The listing builds one solid part. Answer for the finished solid, in the listing's coordinates (mm). Round coordinates to 2 decimals unless told otherwise and drop trailing zeros. Order: outer loops, then holes, each group sorted by start corner. A loop starts at its lowest first (then second) coordinate and runs counter-clockwise, first axis right, second up. Notation, with made-up numbers: M 43.25,-12 L 52.25,-12 A19 cw 52.25,-4 Z; hole C -33,87.5 d3. An arc over 180 degrees is marked long. Put each result on its own line as item: value. Start each with the question number.
1. The part is cut by section D-D (y = -11). Give the vertices of the cut face in (x, z).
2. The part is cut by section A-A (x = -17.5). Give the vertices of the cut face in (y, z).
3. Each of these flat-tipped pins is pushed along its axis until it touches: pin 1 Ø2 at (y, z) = (6, 3.5) entering from -X; pin 2 Ø4 at (y, z) = (4, 6) entering from +X; pin 3 Ø1.1 at (y, z) = (-31, 2.5) entering from +X; pin 4 Ø1.6 at (x, z) = (-2.5, 1.5) entering from +Y. Where does it stop, or does it pass through?
4. The part is cut by section C-C (x = 5). Give the vertices of the cut face in (y, z), then the cut area to 3 significant figures.
5. The part is cut by section B-B (y = -27). Give the vertices of the cut face in (x, z), then the cut area to 3 significant figures.
6. Consider line 1 (Y direction, x = -5, z = 1); line 2 (Y direction, x = 40.48, z = 2.2); line 3 (X direction, y = -54.5, z = 2.25). Determine where each line is inside the solid, lowest interval first.
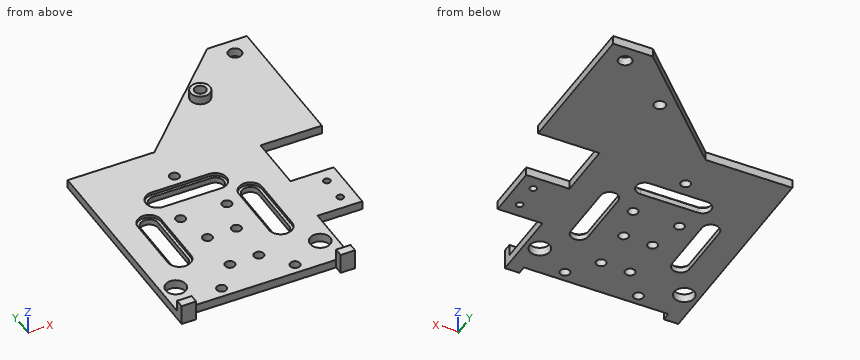
from build123d import *

# Parameters (mm, degrees)
SKETCH_R        = 2.3
SKETCH_R_2      = 1.7
SKETCH_R_3      = 1.2
PAD_DEPTH       = 3
SKETCH004_R     = 2.345013
SKETCH004_R_2   = 1.7
POCKET004_DEPTH = 5
SKETCH003_R     = 3.5
SKETCH003_R_2   = 2
POCKET005_DEPTH = 5
SKETCH005_R     = 3.4
PAD001_DEPTH    = 3
SKETCH006_R     = 2
POCKET_DEPTH    = 8
SKETCH009_R     = 2
POCKET007_DEPTH = 3
POCKET008_DEPTH = 1
SKETCH011_W     = 5
SKETCH011_H     = 3
PAD003_DEPTH    = 3
SKETCH012_W     = 5
SKETCH012_H     = 3
PAD004_DEPTH    = 4


with BuildPart() as part:
    # Sketch → Pad (new body)
    with BuildSketch(Plane.XY):
        Polygon((30, -63), (-30, -63), (-30, 10), (0, 10), (38, 48), (51.73, 48), (51.73, -2), (30.48, -2), (30.48, -22), (45.48, -22), (45.48, -41), (30, -41), align=None)
        with Locations((44.585025, 42.218019)):
            Circle(SKETCH_R, mode=Mode.SUBTRACT)
        with Locations((-12.71, -59.3)):
            Circle(SKETCH_R_2, mode=Mode.SUBTRACT)
        with Locations((12.71, -59.3)):
            Circle(SKETCH_R_2, mode=Mode.SUBTRACT)
        with Locations((0, -3.331213)):
            Circle(SKETCH_R_2, mode=Mode.SUBTRACT)
        with Locations((-8, -22.917882)):
            Circle(SKETCH_R_2, mode=Mode.SUBTRACT)
        with Locations((8, -22.917882)):
            Circle(SKETCH_R_2, mode=Mode.SUBTRACT)
        with Locations((40.48, -27)):
            Circle(SKETCH_R_3, mode=Mode.SUBTRACT)
        with Locations((40.48, -36)):
            Circle(SKETCH_R_3, mode=Mode.SUBTRACT)
        with Locations((-5, -35)):
            Circle(SKETCH_R_2, mode=Mode.SUBTRACT)
        with Locations((5, -35)):
            Circle(SKETCH_R_2, mode=Mode.SUBTRACT)
        with Locations((-5, -50)):
            Circle(SKETCH_R_2, mode=Mode.SUBTRACT)
        with Locations((5, -50)):
            Circle(SKETCH_R_2, mode=Mode.SUBTRACT)
        with BuildLine():
            ThreePointArc((-20.5, -40.385975), (-17.5, -43.385975), (-14.5, -40.385975))
            Line((-14.5, -40.385975), (-14.5, -20.385975))
            ThreePointArc((-14.5, -20.385975), (-17.5, -17.385975), (-20.5, -20.385975))
            Line((-20.5, -40.385975), (-20.5, -20.385975))
        make_face(mode=Mode.SUBTRACT)
        with BuildLine():
            ThreePointArc((14.5, -40.385975), (17.5, -43.385975), (20.5, -40.385975))
            Line((20.5, -40.385975), (20.5, -20.385975))
            ThreePointArc((20.5, -20.385975), (17.5, -17.385975), (14.5, -20.385975))
            Line((14.5, -40.385975), (14.5, -20.385975))
        make_face(mode=Mode.SUBTRACT)
        with BuildLine():
            ThreePointArc((-10, -8.267137), (-13, -11.267137), (-10, -14.267137))
            Line((-10, -14.267137), (10, -14.267137))
            ThreePointArc((10, -14.267137), (13, -11.267137), (10, -8.267137))
            Line((-10, -8.267137), (10, -8.267137))
        make_face(mode=Mode.SUBTRACT)
    extrude(amount=PAD_DEPTH)

    # Sketch004 → Pocket004 (cut)
    with BuildSketch(Plane.XY):
        with Locations((-5, -35)):
            Circle(SKETCH004_R)
        with Locations((-5, -35)):
            Circle(SKETCH004_R_2, mode=Mode.SUBTRACT)
        with Locations((5, -35)):
            Circle(SKETCH004_R_2)
        with Locations((5, -50)):
            Circle(SKETCH004_R_2)
        with Locations((-5, -50)):
            Circle(SKETCH004_R_2)
    extrude(amount=-POCKET004_DEPTH, mode=Mode.SUBTRACT)

    # Sketch003 → Pocket005 (cut)
    with BuildSketch(Plane.XY.offset(3)):
        with Locations((-25, -52.39)):
            Circle(SKETCH003_R)
        with Locations((25, -52.39)):
            Circle(SKETCH003_R)
        with Locations((25, 27.61)):
            Circle(SKETCH003_R_2)
    extrude(amount=-POCKET005_DEPTH, mode=Mode.SUBTRACT)

    # Sketch005 (on Face5 of Pocket005) → Pad001 (join)
    with BuildSketch(Plane.XY.offset(3)):
        with Locations((25, 27.61)):
            Circle(SKETCH005_R)
    extrude(amount=PAD001_DEPTH)

    # Sketch006 (on Face45 of Pad001) → Pocket (cut)
    with BuildSketch(Plane.XY.offset(6)):
        with Locations((25, 27.61)):
            Circle(SKETCH006_R)
    extrude(amount=-POCKET_DEPTH, mode=Mode.SUBTRACT)

    # Sketch009 → Pocket007 (cut)
    with BuildSketch(Plane.XY.offset(4.5)):
        with Locations((25, 27.61)):
            Circle(SKETCH009_R)
    extrude(amount=-POCKET007_DEPTH, mode=Mode.SUBTRACT)

    # Sketch010 (on Face5 of Pocket007) → Pocket008 (cut)
    with BuildSketch(Plane.XY.offset(3)):
        with BuildLine():
            ThreePointArc((-13.5, -20.385975), (-17.5, -16.385975), (-21.5, -20.385975))
            Line((-21.5, -20.385975), (-21.5, -40.385975))
            ThreePointArc((-21.5, -40.385975), (-17.5, -44.385975), (-13.5, -40.385975))
            Line((-13.5, -20.385975), (-13.5, -40.385975))
        make_face()
        with BuildLine():
            ThreePointArc((-10, -7.267137), (-14, -11.267137), (-10, -15.267137))
            Line((-10, -15.267137), (10, -15.267137))
            ThreePointArc((10, -15.267137), (14, -11.267137), (10, -7.267137))
            Line((-10, -7.267137), (10, -7.267137))
        make_face()
        with BuildLine():
            ThreePointArc((21.5, -20.385975), (17.5, -16.385975), (13.5, -20.385975))
            Line((13.5, -20.385975), (13.5, -40.385975))
            ThreePointArc((13.5, -40.385975), (17.5, -44.385975), (21.5, -40.385975))
            Line((21.5, -20.385975), (21.5, -40.385975))
        make_face()
    extrude(amount=-POCKET008_DEPTH, mode=Mode.SUBTRACT)

    # Sketch011 (on Face13 of Pocket008) → Pad003 (join)
    with BuildSketch(Plane.XZ.offset(63)):
        with Locations((-27.5, 1.5)):
            Rectangle(SKETCH011_W, SKETCH011_H)
        with Locations((27.5, 1.5)):
            Rectangle(SKETCH011_W, SKETCH011_H)
    extrude(amount=PAD003_DEPTH)

    # Sketch012 (on Face45 of Pad003) → Pad004 (join)
    with BuildSketch(Plane.XY.offset(3)):
        with Locations((-27.5, -64.5)):
            Rectangle(SKETCH012_W, SKETCH012_H)
        with Locations((27.5, -64.5)):
            Rectangle(SKETCH012_W, SKETCH012_H)
    extrude(amount=PAD004_DEPTH)


solid = part.part
Resolved:
1. outline: M -30,0 L -12.99,0 L -12.99,2 L -13.99,2 L -13.99,3 L -30,3 Z; M 12.99,0 L 30.48,0 L 30.48,3 L 13.99,3 L 13.99,2 L 12.99,2 Z
2. outline: M -63,0 L -43.39,0 L -43.39,2 L -44.39,2 L -44.39,3 L -63,3 Z; M -17.39,0 L 10,0 L 10,3 L -16.39,3 L -16.39,2 L -17.39,2 Z
3. pin 1: x = -30
3. pin 2: through
3. pin 3: x = 45.48
3. pin 4: y = 10
4. outline: M -63,0 L -51.7,0 L -51.7,3 L -63,3 Z; M -48.3,0 L -36.7,0 L -36.7,3 L -48.3,3 Z; M -33.3,0 L -14.27,0 L -14.27,2 L -15.27,2 L -15.27,3 L -33.3,3 Z; M -8.27,0 L 15,0 L 15,3 L -7.27,3 L -7.27,2 L -8.27,2 Z
4. area: 194 mm2
5. outline: M -30,0 L -20.5,0 L -20.5,2 L -21.5,2 L -21.5,3 L -30,3 Z; M -14.5,0 L 14.5,0 L 14.5,2 L 13.5,2 L 13.5,3 L -13.5,3 L -13.5,2 L -14.5,2 Z; M 20.5,0 L 39.28,0 L 39.28,3 L 21.5,3 L 21.5,2 L 20.5,2 Z; M 41.68,0 L 45.48,0 L 45.48,3 L 41.68,3 Z
5. area: 179 mm2
6. line 1: -63 to -51.7, -48.3 to -36.7, -33.3 to -14.27, -8.27 to 10
6. line 2: -41 to -37.2, -34.8 to -28.2, -25.8 to -22, -2 to 48
6. line 3: -30 to -27.79, -22.21 to 22.21, 27.79 to 30
